```python
from build123d import *

# Parameters (mm, degrees)
ESQUISSE1_W             = 10
ESQUISSE1_H             = 41.761471848
ESQUISSE1_W_2           = 20
ESQUISSE1_H_2           = 11.28355545
BOSS_EXTRU_1_DEPTH      = 20
CONG_1_R                = 20
ESQUISSE2_R             = 4.9
BOSS_EXTRU_2_DEPTH      = 10
ESQUISSE4_W             = 62.840930267
ESQUISSE4_H             = 35.08297334
ENL_V_MAT_EXTRU_1_DEPTH = 10
ESQUISSE6_R             = 3.25
BOSS_EXTRU_3_DEPTH      = 9


with BuildPart() as part:
    # Esquisse1 → Boss.-Extru.1 (new body)
    with BuildSketch(Plane.XY):
        Polygon((0, 0), (0, 21.28355545), (-40, 21.28355545), (-110, 46.761471848), (-110, 61.761471848), (-130, 61.761471848), (-130, 0), (-110, 0), (-110, 25.477916399), (-40, 0), align=None)
        Polygon((-107.5, 40.5306574), (-45, 17.782517758), (-45, 7.140740034), (-107.5, 29.888879675), align=None, mode=Mode.SUBTRACT)
        with Locations((-120, 25.880735924)):
            Rectangle(ESQUISSE1_W, ESQUISSE1_H, mode=Mode.SUBTRACT)
        with Locations((-25, 10.641777725)):
            Rectangle(ESQUISSE1_W_2, ESQUISSE1_H_2, mode=Mode.SUBTRACT)
    extrude(amount=BOSS_EXTRU_1_DEPTH)

    # Congé1
    cong_1_edges = [part.edges().sort_by_distance(p)[0] for p in [
        (-110, 46.761471848, 10),
    ]]
    fillet(cong_1_edges, radius=CONG_1_R)

    # Esquisse2 → Boss.-Extru.2 (add)
    with BuildSketch(Plane(origin=(0, 61.761471848, 0), x_dir=(1, 0, 0), z_dir=(0, 1, 0))):
        with Locations(Location((-120, -10, 0), (0, 0, 270))):
            Circle(ESQUISSE2_R)
    extrude(amount=BOSS_EXTRU_2_DEPTH)

    # Esquisse4 → Enlèv. mat.-Extru.1 (cut)
    with BuildSketch(Plane(origin=(0, 0, 0), x_dir=(0, 0, -1), z_dir=(1, 0, 0))):
        with Locations((-15.686525899, 12.319682914)):
            Rectangle(ESQUISSE4_W, ESQUISSE4_H)
    extrude(amount=-ENL_V_MAT_EXTRU_1_DEPTH, mode=Mode.SUBTRACT)

    # Esquisse6 → Boss.-Extru.3 (add)
    with BuildSketch(Plane(origin=(-10, 0, 0), x_dir=(0, 0, -1), z_dir=(1, 0, 0))):
        with Locations((-15, 10.641777725)):
            Circle(ESQUISSE6_R)
        with Locations(Location((-5, 10.641777725, 0), (0, 0, 180))):
            Circle(ESQUISSE6_R)
    extrude(amount=BOSS_EXTRU_3_DEPTH)


solid = part.part
```
Geometry check sheet. Reference: the model listing, model coordinates, mm. A direction names the side the tool comes from. Round coordinates to 2 decimals unless told otherwise and drop trailing zeros. Write each loop counter-clockwise with the first axis right and the second up, starting at its lowest first coordinate (ties: lowest second). Pieces come first, ordered by that corner, then holes. Notation, with made-up numbers: (69, -29.5) - (73, -29.5) arc R10 ccw to (73, -11.5) - close; hole circle Ø6 at (58.5, 30.5). An arc over 180 degrees is marked (long way). Write each question's results on one line, items separated by ' | '.
(1) Sectioned sample at B-B, the plane z = 10. Enter the section's corners in (x, y).
Computed:
outline: (-130, 0) - (-110, 0) - (-110, 25.48) - (-40, 0) - (-10, 0) - (-10, 21.28) - (-40, 21.28) - (-96.84, 41.97) arc R20 cw to (-110, 60.77) - (-110, 61.76) - (-115.1, 61.76) - (-115.1, 71.76) - (-124.9, 71.76) - (-124.9, 61.76) - (-130, 61.76) - close; hole (-125, 5) - (-115, 5) - (-115, 46.76) - (-125, 46.76) - close; hole (-107.5, 29.89) - (-45, 7.14) - (-45, 17.78) - (-107.5, 40.53) - close; hole (-35, 5) - (-15, 5) - (-15, 16.28) - (-35, 16.28) - close
(2) Set-up check for faces 1 (the face through (-118, 61.761, 5)), 2 (the face through (-130, 31, 10)), 3 (the face through (-5.563, 13.525, 6.5)), 4 (the face through (-125, 26, 10)): record each of +Z, -Z, +X, -X, +Y, -Y from which the full face is reachable in a straight line by a thin tool's end or side.
Computed:
face 1: +Y | face 2: +Z, -Z, -X, +Y, -Y | face 3: +X | face 4: +Z, -Z
(3) Depth check by flat-ended pin: pin 1 Ø3 at (x, z) = (-99.5, 7) entering from +Y; pin 2 Ø0.8 at (y, z) = (61, 8) entering from +X; pin 3 Ø8 at (x, z) = (-57, 11) entering from +Y. Enter the tip coordinate at first touch or a pass-through.
Computed:
pin 1: stops at y = 44.06 | pin 2: stops at x = -110 | pin 3: stops at y = 28.93
(4) Sectioned sample at D-D, the plane y = 36. Enter the section's corners in (x, z), plus the area to 3 significant figures.
Computed:
outline: (-130, 0) - (-125, 0) - (-125, 20) - (-130, 20) - close; (-115, 0) - (-107.5, 0) - (-107.5, 20) - (-115, 20) - close; (-95.05, 0) - (-80.43, 0) - (-80.43, 20) - (-95.05, 20) - close | area: 542 mm^2
(5) Draft check along X on faces 5 (the face through (-25, 0, 10)), 6 (the face through (-10, 11, 10)), 7 (the face through (-115, 26, 10)). Enter one of: pulls with the +X half, pulls with the -X half, needs draft (parallel to the pull), parting line crosses it, or undercut.
Computed:
face 5: needs draft | face 6: pulls with the +X half | face 7: undercut
(6) Thickness scan on probe 1 along Y at (x, z) = (-33.5, 6); probe 2 along Y at (x, z) = (-118.5, 5.5); probe 3 along X at (y, z) = (45.5, 4). Record the ranges inside material, lowest first. Write a range as from..to.
Computed:
probe 1: y = 0..5, 16.28..21.28 | probe 2: y = 0..5, 46.76..71.76 | probe 3: x = -130..-125, -115..-102.92
(7) Sectioned sample at C-C, the plane y = 23. Enter the section's corners in (x, z).
Computed:
outline: (-130, 0) - (-125, 0) - (-125, 20) - (-130, 20) - close; (-115, 0) - (-110, 0) - (-110, 20) - (-115, 20) - close; (-103.19, 0) - (-88.57, 0) - (-88.57, 20) - (-103.19, 20) - close; (-59.33, 0) - (-44.72, 0) - (-44.72, 20) - (-59.33, 20) - close
(8) Sectioned sample at A-A, the plane x = -30. Enter the section's corners in (y, z), plus the area to 3 significant figures.
Computed:
outline: (0, 0) - (5, 0) - (5, 20) - (0, 20) - close; (16.28, 0) - (21.28, 0) - (21.28, 20) - (16.28, 20) - close | area: 200 mm^2
